```python
from build123d import *
from build123d.topology import SkipClean

# Parameters (mm, degrees)
BOSS_EXTRUDE1_DEPTH       = 4
M3X0_5_TAPPED_HOLE1_D     = 2.5
M3X0_5_TAPPED_HOLE1_DEPTH = 7.5
M3X0_5_TAPPED_HOLE1_TIP   = 0.751075774
SKETCH5_R                 = 1.25
BOSS_EXTRUDE2_DEPTH       = 5


with BuildPart() as part:
    # Sketch1 → Boss-Extrude1 (new body)
    with BuildSketch(Plane.XY):
        Polygon((0, 2.886751346), (-2.5, 1.443375673), (-2.5, -1.443375673), (0, -2.886751346), (2.5, -1.443375673), (2.5, 1.443375673), align=None)
    extrude(amount=BOSS_EXTRUDE1_DEPTH)

    # M3x0.5 Tapped Hole1
    with Locations(Plane.XY.offset(4)):
        with Locations((0, 0)):
            Hole(M3X0_5_TAPPED_HOLE1_D / 2, depth=M3X0_5_TAPPED_HOLE1_DEPTH)
            with Locations((0, 0, -(M3X0_5_TAPPED_HOLE1_DEPTH + M3X0_5_TAPPED_HOLE1_TIP / 2))):  # 118° drill point
                Cone(0, M3X0_5_TAPPED_HOLE1_D / 2, M3X0_5_TAPPED_HOLE1_TIP, mode=Mode.SUBTRACT)

    # Sketch4 → Cut-Revolve1 (revolve, cut)
    with BuildSketch(Plane(origin=(0, 0, 0), x_dir=(0, 0, -1), z_dir=(1, 0, 0)), mode=Mode.PRIVATE) as cut_revolve1_sk:
        Polygon((-3.776709006, 2.886751346), (-4, 2.5), (-4, 2.886751346), align=None)
        Polygon((0, 2.886751346), (-0.223290994, 2.886751346), (0, 2.5), align=None)
    revolve(cut_revolve1_sk.sketch.rotate(Axis((0, 0, 0), (0, 0, 1)), 270), axis=Axis((0, 0, 0), (0, 0, 1)), mode=Mode.SUBTRACT)

    # Sketch5 → Boss-Extrude2 (add)
    with SkipClean():  # the faces are left unmerged after this step: merging them gives an invalid solid
        with BuildSketch(Plane.XY.offset(4)):
            with BuildLine():
                ThreePointArc((1.25, -2.165063509), (2.165063509, -1.25), (2.5, 0))
                ThreePointArc((2.5, 0), (2.165063509, 1.25), (1.25, 2.165063509))
                ThreePointArc((1.25, 2.165063509), (0, 2.5), (-1.25, 2.165063509))
                ThreePointArc((-1.25, 2.165063509), (-2.165063509, 1.25), (-2.5, 0))
                ThreePointArc((-2.5, 0), (-2.165063509, -1.25), (-1.25, -2.165063509))
                ThreePointArc((-1.25, -2.165063509), (0, -2.5), (1.25, -2.165063509))
            make_face()
            Circle(SKETCH5_R, mode=Mode.SUBTRACT)
        extrude(amount=BOSS_EXTRUDE2_DEPTH)
    add(part.part.scale(1), mode=Mode.REPLACE)  # the faces are merged on a copy


solid = part.part
```
Check sheet for the modelled part. Datum: model origin and axes. Units: mm. Coordinates: 2 decimals unless noted, no trailing zeros. Loops run counter-clockwise (first coordinate to the right, second up) from the corner with the lowest first, then second, coordinate; pieces in that order, holes last.
1) Material ranges on probe 1 along Y at (x, z) = (0, 5.55); probe 2 along Y at (x, z) = (-0.9, 6.25), recorded low to high.
2) Gauge pin test, flat ends, axial feed: pin 1 (3 mm diameter, centred on x = 0, y = 0, fed in from -Z); pin 2 (1.5 mm diameter, centred on x = -1, z = 6, fed in from +Y). Record the tip position at first contact, or that the pin passes through.
3) Sectioned sample at B-B (z = 6.5). Record the boundary of the cut face in (x, y), and give its area (3 significant figures).
4) Sectioned sample at A-A (z = 2.5). Record the boundary of the cut face in (x, y), and give its area (3 significant figures).
Check sheet entries:
1. probe 1: y = -2.5 to -1.25, 1.25 to 2.5
1. probe 2: y = -2.33 to -0.87, 0.87 to 2.33
2. pin 1: stops at z = 0
2. pin 2: stops at y = 2.49
3. outline: circle Ø5 at (0, 0); hole circle Ø2.5 at (0, 0)
3. area: 14.7 mm2
4. outline: (-2.5, -1.44) - (0, -2.89) - (2.5, -1.44) - (2.5, 1.44) - (0, 2.89) - (-2.5, 1.44) - close; hole circle Ø2.5 at (0, 0)
4. area: 16.7 mm2
